```python
from build123d import *

# Parameters (mm, degrees)
F1_DEPTH      = 63.5
F1_DEPTH_BACK = 63.5
F2_W          = 121.412
F2_H          = 121.4773469555
F3_DEPTH      = 10.16
F6_ANGLE_BACK = 4.9623752699
F6_ANGLE      = 9.6002572001


with BuildPart() as f1:
    # F0 (on Right) → F1 (new body, two sides)
    with BuildSketch(Plane.YZ) as f1_sk:
        with BuildLine():
            Line((-44.2258762484, -5.1661990916), (-45.3097894054, -15.0418539721))
            ThreePointArc((-45.3097894054, -15.0418539721), (-13.7030518217, -21.9890417418), (18.6550981372, -21.5424884693))
            ThreePointArc((18.6550981372, -21.5424884693), (47.8654596913, -23.2074448835), (75.9852901101, -15.1270711794))
            Line((75.9852901101, -15.1270711794), (76.2974227243, -12.2831957683))
            Line((76.2974227243, -12.2831957683), (81.7933529615, -9.5837377012))
            Line((81.7933529615, -9.5837377012), (81.7933529615, 3.07087185))
            ThreePointArc((81.7933529615, 3.07087185), (83.9552126708, 4.627317683), (86.0872641206, 6.2243516994))
            Line((86.0872641206, 6.2243516994), (86.0872641206, 63.1598830223))
            Line((86.0872641206, 63.1598830223), (64.0061274171, 65.0746673346))
            ThreePointArc((64.0061274171, 65.0746673346), (58.5946758607, 66.3143740435), (54.1078224778, 69.5837512612))
            ThreePointArc((54.1078224778, 69.5837512612), (15.5800187481, 99.1361263011), (-31.4539738675, 111.2000423056))
            Line((-31.4539738675, 111.2000423056), (-43.6588544929, 0))
            Line((-43.6588544929, 0), (-38.2017120719, 0))
            Line((-38.2017120719, 0), (-38.7687338274, -5.1661990916))
            Line((-38.7687338274, -5.1661990916), (-44.2258762484, -5.1661990916))
        make_face()
        Polygon((-43.6588544929, 0), (-44.2258762484, -5.1661990916), (-38.7687338274, -5.1661990916), (-38.2017120719, 0), align=None)
    extrude(amount=F1_DEPTH)
    extrude(f1_sk.sketch, amount=-F1_DEPTH_BACK)

    # F2 (on face) → F3 (cut)
    with BuildSketch(Plane(origin=(0, -43.1391827765, 4.7347875518), x_dir=(1, 0, 0), z_dir=(0, -0.9940306794, 0.1091009097))):
        with Locations((0, 43.5864519963)):
            Rectangle(F2_W, F2_H)
    extrude(amount=-F3_DEPTH, mode=Mode.SUBTRACT)

    # F5 (on offset) → F6 (revolve)
    with BuildSketch(Plane(origin=(0, 4.4781674488, 40.8010881091), x_dir=(1, 0, 0), z_dir=(0, -0.1091009097, -0.9940306794)), mode=Mode.PRIVATE) as f6_sk:
        with BuildLine():
            ThreePointArc((63.1147550677, 37.2976302589), (0, 40.7020876312), (-63.1147550677, 37.2976302589))
            Line((-63.1147550677, 37.2976302589), (63.1147550677, 37.2976302589))
        make_face()
    revolve(f6_sk.sketch.rotate(Axis((60.319211334, 698.4784697554, -35.36966388), (1, 0, 0)), -F6_ANGLE_BACK), axis=Axis((60.319211334, 698.4784697554, -35.36966388), (1, 0, 0)), revolution_arc=F6_ANGLE)


solid = f1.part
```
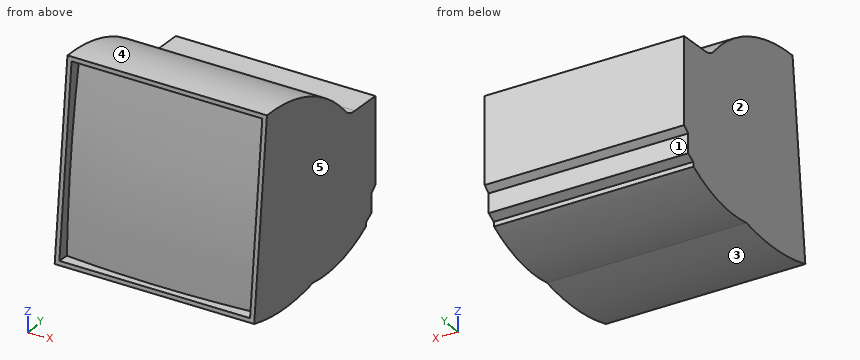
The listing builds one solid part. Answer for the finished solid, in the listing's coordinates (mm). Face numbers are marked on the shaded views. A direction names the side the tool comes from. Give positions to 0.01 mm unless a question says otherwise; leave off trailing zeros. Loops run counter-clockwise (first coordinate to the right, second up) from the corner with the lowest first, then second, coordinate; pieces in that order, holes last. Notation, with made-up numbers: M 53,-14.75 L 73,-14.75 A18 ccw 73,6.25 Z; hole C 68,-25.5 d3. An arc over 180 degrees is marked long. One line per item, written item: value.
1. For a pull along Y with two mould halves and no side action, classify the marked faces 3, 4 and 5 as pulls with the +Y half, pulls with the -Y half, needs draft (parallel to the pull), parting line crosses it, or undercut.
Found:
face 3: undercut
face 4: pulls with the +Y half
face 5: needs draft
2. Find the intervals of material crossed by probe 1 along X at (y, z) = (-36, 66.5); probe 2 along Y at (x, z) = (-30, 36); probe 3 along Y at (x, z) = (-53, 95.5), in increasing order.
Found:
probe 1: -63.5 to -60.71, 60.71 to 63.5
probe 2: -36.17 to -33.52, -29.49 to 86.09
probe 3: -26.27 to -25.25, -22.96 to 22.48
3. Each of these flat-tipped pins is pushed along its axis until it touches: P1, Ø3, axis at x = -12, z = 26, coming from the -Y side; P2, Ø6, axis at x = 6, y = -3.5, coming from the +Z side; P3, Ø12, axis at x = -33.5, y = 11.5, coming from the +Z side. Where does it stop, or does it pass through?
Found:
P1: y = -37.84
P2: z = 107.33
P3: z = 103.49
4. Section B-B on y = 61 is taken. Determine the outline of the cut face in (x, z), plus the area to 3 significant figures.
Found:
outline: M -63.5,-20.71 L 63.5,-20.71 L 63.5,65.48 L -63.5,65.48 Z
area: 10,900 mm^2
5. Section A-A on y = -26.5 is taken. State how many separate pieces and enclosed holes the cut face has, plus the area to 3 significant figures.
Found:
separate pieces: 1
enclosed holes: 2
area: 12,800 mm^2
6. For the marked faces 1 and 2, determine the directions among +Z, -Z, +X, -X, +Y, -Y from which every point of the face is accessible in a straight line to the end or side of a thin tool.
Found:
face 1: -Z, +X, -X, +Y
face 2: +Z, -Z, -X, +Y, -Y
7. Section C-C on y = 4 is taken. Determine the outline of the cut face in (x, z), plus the area to 3 significant figures.
Found:
outline: M -63.5,-22.67 L 63.5,-22.67 L 63.5,104.04 L -63.5,104.04 Z
area: 16,100 mm^2
